```python
from build123d import *

# Parameters (mm, degrees)
SKETCH3_W           = 57.15
SKETCH3_H           = 30.48
BOSS_EXTRUDE2_DEPTH = 3.175
SKETCH4_W           = 57.15
SKETCH4_H           = 3.175
BOSS_EXTRUDE3_DEPTH = 22.225
SKETCH6_R           = 1.25
CUT_EXTRUDE1_DEPTH  = 3.175
SKETCH7_R           = 3.175
CUT_EXTRUDE2_DEPTH  = 3.175


with BuildPart() as part:
    # Sketch3 → Boss-Extrude2 (new body)
    with BuildSketch(Plane.XY):
        with Locations((28.575, 15.24)):
            Rectangle(SKETCH3_W, SKETCH3_H)
    extrude(amount=BOSS_EXTRUDE2_DEPTH)

    # Sketch4 → Boss-Extrude3 (add)
    with BuildSketch(Plane.XY.offset(3.175)):
        with Locations((28.575, 28.8925)):
            Rectangle(SKETCH4_W, SKETCH4_H)
    extrude(amount=BOSS_EXTRUDE3_DEPTH)

    # Sketch6 → Cut-Extrude1 (cut)
    with BuildSketch(Plane(origin=(0, 30.48, 0), x_dir=(1, 0, 0), z_dir=(0, 1, 0))):
        with Locations(Location((36.353174593, -18.1939997, 0), (0, 0, 270))):
            Circle(SKETCH6_R)
        with Locations(Location((20.796825407, -18.1939997, 0), (0, 0, 270))):
            Circle(SKETCH6_R)
    extrude(amount=-CUT_EXTRUDE1_DEPTH, mode=Mode.SUBTRACT)

    # Sketch7 → Cut-Extrude2 (cut)
    with BuildSketch(Plane.XY.offset(3.175)):
        with Locations((47.625, 13.713)):
            Circle(SKETCH7_R)
        with Locations((9.525, 13.713)):
            Circle(SKETCH7_R)
    extrude(amount=-CUT_EXTRUDE2_DEPTH, mode=Mode.SUBTRACT)


solid = part.part
```
The listing builds one solid part. Answer for the finished solid, in the listing's coordinates (mm). A direction names the side the tool comes from. Give positions to 0.01 mm unless a question says otherwise; leave off trailing zeros. Order: outer loops, then holes, each group sorted by start corner. A loop starts at its lowest first (then second) coordinate and runs counter-clockwise, first axis right, second up. Notation, with made-up numbers: (40, -22.5) -> (80, -22.5) arc R35 ccw to (80, 16.5) -> close; hole circle Ø10 at (-14.5, 14). An arc over 180 degrees is marked (long way). Write each question's results on one line, items separated by ' | '.
Q1. The part is cut by section D-D, the plane z = 4.25. Give the vertices of the cut face in (x, y) (3 decimals).
Checked values:
outline: (0, 27.305) -> (57.15, 27.305) -> (57.15, 30.48) -> (0, 30.48) -> close
Q2. The part is cut by section C-C, the plane y = 17.5. Give the vertices of the cut face in (x, z) (3 decimals).
Checked values:
outline: (0, 0) -> (57.15, 0) -> (57.15, 3.175) -> (0, 3.175) -> close
Q3. Each of these flat-tipped pins is pushed along its axis until it touches: P1, Ø3, axis at x = 25, y = 10, coming from the -Z side; P2, Ø5, axis at x = 8.5, y = 15, coming from the +Z side (3 decimals); P3, Ø3, axis at x = 36.35, z = 18.19, coming from the -Y side (3 decimals). Where does it stop, or does it pass through?
Checked values:
P1: stops at z = 0 | P2: stops at z = 3.175 | P3: stops at y = 27.305
Q4. Which of the six approach directions +Z, -Z, +X, -X, +Y, -Y give full straight-line access (tool end or side, diameter ignored) to faces 1 (the face through (0, 21, 2)), 2 (the face through (28, 27.305, 14))?
Checked values:
face 1: +Z, -Z, -X, +Y, -Y | face 2: +Z, +X, -X, -Y
Q5. Determine the mould class of faces 3 (the face through (20.852, 28.915, 16.945)), 4 (the face through (57.15, 21, 2)), 5 (the face through (28, 30.48, 13)) for opening direction X: pulls with the +X half, pulls with the -X half, needs draft (parallel to the pull), parting line crosses it, or undercut.
Checked values:
face 3: undercut | face 4: pulls with the +X half | face 5: needs draft
Q6. Straight lines are drawn through the part: probe 1 along Z at (x, y) = (46.5, 23) (3 decimals); probe 2 along Y at (x, z) = (22.5, 15) (3 decimals). For each, find the intervals that lie inside material, in ascending order. Write a range as from..to.
Checked values:
probe 1: z = 0..3.175 | probe 2: y = 27.305..30.48
Q7. The part is cut by section B-B, the plane z = 18.25. Give the vertices of the cut face in (x, y) (3 decimals).
Checked values:
outline: (0, 27.305) -> (19.548, 27.305) -> (19.548, 30.48) -> (0, 30.48) -> close; (22.046, 27.305) -> (35.104, 27.305) -> (35.104, 30.48) -> (22.046, 30.48) -> close; (37.602, 27.305) -> (57.15, 27.305) -> (57.15, 30.48) -> (37.602, 30.48) -> close
Q8. The part is cut by section A-A, the plane x = 11. Give the vertices of the cut face in (y, z) (3 decimals).
Checked values:
outline: (0, 0) -> (10.901, 0) -> (10.901, 3.175) -> (0, 3.175) -> close; (16.525, 0) -> (30.48, 0) -> (30.48, 25.4) -> (27.305, 25.4) -> (27.305, 3.175) -> (16.525, 3.175) -> close
